```python
from build123d import *

# Parameters (mm, degrees)
SKETCH_W        = 50
SKETCH_H        = 50
PAD_DEPTH       = 10
CHAMFER_SIZE    = 2
CHAMFER001_SIZE = 2


with BuildPart() as part:
    # Sketch → Pad (new body)
    with BuildSketch(Plane.XY):
        Rectangle(SKETCH_W, SKETCH_H)
    extrude(amount=PAD_DEPTH)

    # Chamfer
    chamfer_edges = [part.edges().sort_by_distance(p)[0] for p in [
        (0, -25, 10),
        (25, 0, 10),
    ]]
    chamfer(chamfer_edges, length=CHAMFER_SIZE)

    # Chamfer001
    chamfer001_edges = [part.edges().sort_by_distance(p)[0] for p in [
        (-25, -25, 4),
    ]]
    chamfer(chamfer001_edges, length=CHAMFER001_SIZE)


solid = part.part
```
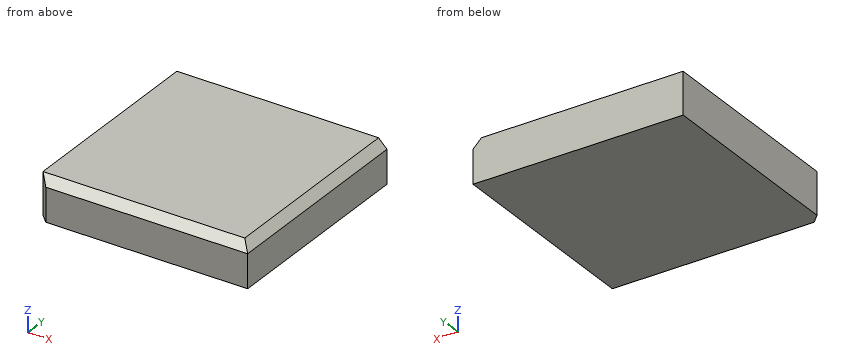
Read the model definition and answer for the solid it produces. Units are mm, in the model's axes. Round coordinates to 2 decimals unless told otherwise and drop trailing zeros. Write each loop counter-clockwise with the first axis right and the second up, starting at its lowest first coordinate (ties: lowest second). Pieces come first, ordered by that corner, then holes. Notation, with made-up numbers: (33.25, -24) - (59.25, -24) arc R21 ccw to (59.25, 4) - close; hole circle Ø7 at (27.25, 49). An arc over 180 degrees is marked (long way). Use CSV: the item, a comma, the result in double quotes.
Q1. This flat-tipped pin is pushed along its axis until it touches: pin 1 Ø10 at (x, y) = (-14, 4.5) entering from -Z. Where does it stop, or does it pass through?
Values:
pin 1,"stops at z = 0"
Q2. Straight lines are drawn through the part: line 1 along X through (y, z) = (-7, 9); line 2 along Y through (x, z) = (4, 9); line 3 along X through (y, z) = (-12, 8.5). For each, find the intervals that lie inside material, in ascending order.
Values:
line 1,"x = -25 to 24"
line 2,"y = -24 to 25"
line 3,"x = -25 to 24.5"
Q3. Find section A-A, the plane z = 9. Write down the section's boundary in (x, y), then the cut area to 3 significant figures.
Values:
outline,"(-25, -23) - (-24, -24) - (24, -24) - (24, 25) - (-25, 25) - close"
area,"2,400 mm²"
